Print and shaded views of the part. All mm, measured from the part's lowest x, y and z. A direction names the side the tool comes from. Give positions to 0.01 mm unless a question says otherwise; leave off trailing zeros. Write each loop counter-clockwise with the first axis right and the second up, starting at its lowest first coordinate (ties: lowest second). Pieces come first, ordered by that corner, then holes. Notation, with made-up numbers: (51.5, 10.25) - (100.5, 10.25) arc R32 cw to (100.5, 47.25) - close; hole circle Ø4 at (-4, 29). An arc over 180 degrees is marked (long way). Use one line per item in the form item = value. Start each with the question number.
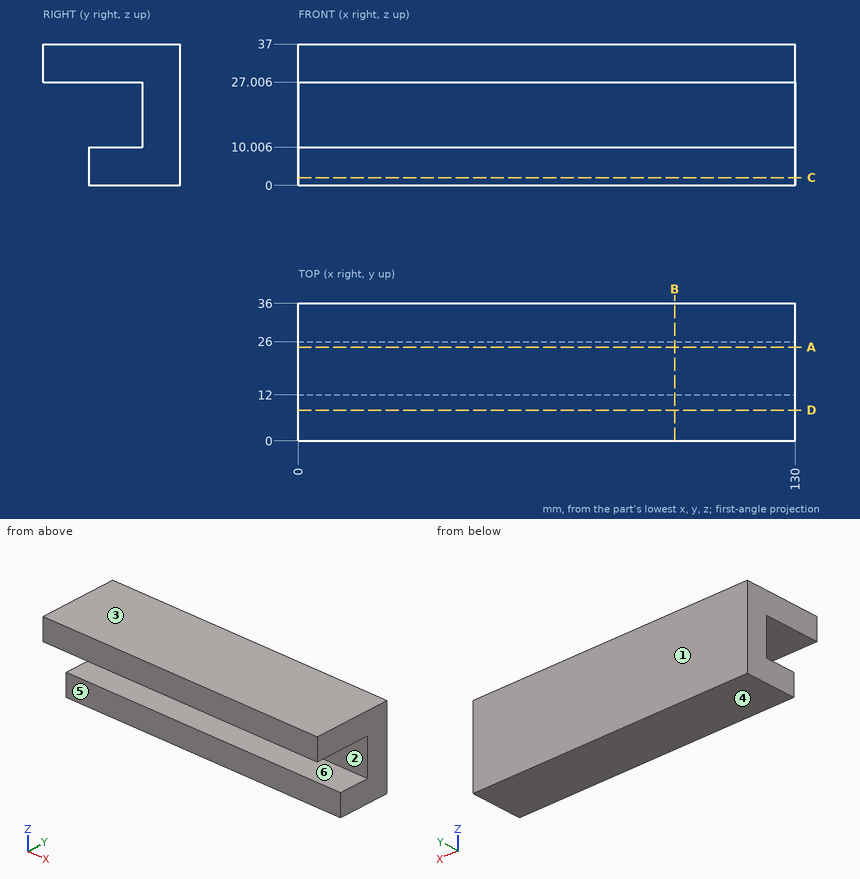
(1) Cut at C-C, the plane z = 2. Give the cut face in (x, y), then the cut area to 3 significant figures.
(2) Cut at A-A, the plane y = 24.5. Give the cut face in (x, z), then the cut area to 3 significant figures.
(3) Which spindle directions (+Z, -Z, +X, -X, +Y, -Y) get a long thin tool onto all of the face, cutting with end or side? Do the marked faces 4, 5 and 6. Say none if no direction does.
(4) Cut at B-B, the plane x = 98.5. Give the cut face in (y, z).
(5) Two-plate mould, pull along Z, no slides. Class the marked faces 1, 2 and 3: +Z half, -Z half, draft (parallel to the pull), parting line (faces both ways), or undercut.
(6) Wall check: line 1 (Z direction, x = 41.5, y = 22); line 2 (Y direction, x = 71, z = 8.5); line 3 (Z direction, x = 117, y = 3.5). Give the ranges that are in metal, low to high. Write a range as from..to.
(7) Pin check, flat tips, straight feed: pin 1 Ø8 at (x, y) = (26.5, 24.5) entering from -Z; pin 2 Ø3 at (x, z) = (112.5, 21) entering from -Y; pin 3 Ø5 at (x, z) = (21, 11) entering from -Y. Stop position of each tip, or through.
(8) Cut at D-D, the plane y = 8. Give the cut face in (x, z).
Solution:
q1.outline = (0, 12) - (130, 12) - (130, 36) - (0, 36) - close
q1.area = 3,120 mm2
q2.outline = (0, 0) - (130, 0) - (130, 10.01) - (0, 10.01) - close; (0, 27.01) - (130, 27.01) - (130, 37) - (0, 37) - close
q2.area = 2,600 mm2
q3.face_4 = -Z, +X, -X, +Y, -Y
q3.face_5 = -Z, +X, -X, -Y
q3.face_6 = +X, -X, -Y
q4.outline = (0, 27.01) - (26, 27.01) - (26, 10.01) - (12, 10.01) - (12, 0) - (36, 0) - (36, 37) - (0, 37) - close
q5.face_1 = draft
q5.face_2 = undercut
q5.face_3 = +Z half
q6.line_1 = 0..10.01, 27.01..37
q6.line_2 = 12..36
q6.line_3 = 27.01..37
q7.pin_1 = 0
q7.pin_2 = 26
q7.pin_3 = 12
q8.outline = (0, 27.01) - (130, 27.01) - (130, 37) - (0, 37) - close
